For this review, take the finished solid that the model builds, in its own axes (mm). A direction names the side the tool comes from. Give positions to 0.01 mm unless a question says otherwise; leave off trailing zeros. Loops run counter-clockwise (first coordinate to the right, second up) from the corner with the lowest first, then second, coordinate; pieces in that order, holes last. Notation, with made-up numbers: M -7,65 L 28,65 A18 ccw 28,77 Z; hole C 72,-9 d8. An arc over 180 degrees is marked long. Use CSV: the item, a comma, the result in double quotes. Start each with the question number.
1. Take a section at C-C, the plane y = 44. Write out the cut boundary in (x, z), and give its area (3 significant figures).
2. Insertion check: P1, Ø2.5, axis at x = 4.76, y = -11.56, coming from the -Z side; P2, Ø6, axis at x = 11, y = 50.86, coming from the -Z side; P3, Ø3, axis at x = 37, z = 70, coming from the -Y side; P4, Ø5, axis at y = 14, z = 74.5, coming from the +X side. Each pin has a flat end and moves straight along its axis. Give the tip position at first contact, or say it passes through.
3. Tool access review of faces 3 (the face through (-6, -11, 75.5)), 4 (the face through (6.146, -11.121, 72.712)), 5 (the face through (0, -5, 70)): name each direction out of +Z, -Z, +X, -X, +Y, -Y from which nothing blocks a thin tool from reaching the whole face with its end or side.
4. The part is to be moulded in two halves that separate along X. For faces 1 (the face through (28, 1, 70)), 2 (the face through (9.214, -52.229, 73.944)), say which applies: pulls with the +X half, pulls with the -X half, needs draft (parallel to the pull), parting line crosses it, or undercut.
5. Take a section at D-D, the plane x = -36.5. Write out the cut boundary in (y, z), and give its area (3 significant figures).
6. Take a section at B-B, the plane z = 72. State how many separate pieces and enclosed holes the cut face has, and give its area (3 significant figures).
7. To check wall thickness, follow line 1 (Y direction, x = -11, z = 76.25); line 2 (Y direction, x = -11.5, z = 71.75); line 3 (Z direction, x = 26, y = -57.5). State the ranges of each line that lie inside material, in increasing order. Write a range as [from, to].
8. Take a section at A-A, the plane x = 0. Write out the cut boundary in (y, z).
from build123d import *

# Parameters (mm, degrees)
DISCO_START                         = 70
SK_DISCO_R                          = 65
DISCO_DEPTH                         = 8
CENTRADOR_ARANDELA_EJE_51110_START  = 67
SK_CENTRADOR_ARANDELA_EJE_51110_R   = 24.9
SK_CENTRADOR_ARANDELA_EJE_51110_R_2 = 23
CENTRADOR_ARANDELA_EJE_51110_DEPTH  = 3
PASANTES_M2_5_ROTOR_J1_START        = 70
SK_PASANTES_M2_5_ROTOR_J1_R         = 1.45
PASANTES_M2_5_ROTOR_J1_DEPTH        = 8
CAJAS_M2_5_START                    = 75.5
SK_CAJAS_M2_5_R                     = 2.75
CAJAS_M2_5_DEPTH                    = 2.5
PASO_CABLE_START                    = 70
SK_PASO_CABLE_R                     = 3
PASO_CABLE_DEPTH                    = 8
PASANTES_M4_ANGULOS_START           = 70
SK_PASANTES_M4_ANGULOS_R            = 2.25
PASANTES_M4_ANGULOS_DEPTH           = 8


with BuildPart() as part:
    # Sk_Disco → Disco (new body)
    with BuildSketch(Plane.XY.offset(DISCO_START)):
        Circle(SK_DISCO_R)
    extrude(amount=DISCO_DEPTH)

    # Sk_Centrador_arandela_eje_51110 → Centrador_arandela_eje_51110 (add)
    with BuildSketch(Plane.XY.offset(CENTRADOR_ARANDELA_EJE_51110_START)):
        Circle(SK_CENTRADOR_ARANDELA_EJE_51110_R)
        Circle(SK_CENTRADOR_ARANDELA_EJE_51110_R_2, mode=Mode.SUBTRACT)
    extrude(amount=CENTRADOR_ARANDELA_EJE_51110_DEPTH)

    # Sk_Pasantes_M2-5_rotor_J1 → Pasantes_M2-5_rotor_J1 (cut)
    with BuildSketch(Plane.XY.offset(PASANTES_M2_5_ROTOR_J1_START)):
        with Locations((12.390194253, -1.653204878)):
            Circle(SK_PASANTES_M2_5_ROTOR_J1_R)
        with Locations((7.626814549, 9.903620542)):
            Circle(SK_PASANTES_M2_5_ROTOR_J1_R)
        with Locations((-4.763379704, 11.55682542)):
            Circle(SK_PASANTES_M2_5_ROTOR_J1_R)
        with Locations((-12.390194253, 1.653204878)):
            Circle(SK_PASANTES_M2_5_ROTOR_J1_R)
        with Locations((-7.626814549, -9.903620542)):
            Circle(SK_PASANTES_M2_5_ROTOR_J1_R)
        with Locations((4.763379704, -11.55682542)):
            Circle(SK_PASANTES_M2_5_ROTOR_J1_R)
    extrude(amount=PASANTES_M2_5_ROTOR_J1_DEPTH, mode=Mode.SUBTRACT)

    # Sk_Cajas_M2-5 → Cajas_M2-5 (cut)
    with BuildSketch(Plane.XY.offset(CAJAS_M2_5_START)):
        with Locations((12.390194253, -1.653204878)):
            Circle(SK_CAJAS_M2_5_R)
        with Locations((7.626814549, 9.903620542)):
            Circle(SK_CAJAS_M2_5_R)
        with Locations((-4.763379704, 11.55682542)):
            Circle(SK_CAJAS_M2_5_R)
        with Locations((-12.390194253, 1.653204878)):
            Circle(SK_CAJAS_M2_5_R)
        with Locations((-7.626814549, -9.903620542)):
            Circle(SK_CAJAS_M2_5_R)
        with Locations((4.763379704, -11.55682542)):
            Circle(SK_CAJAS_M2_5_R)
    extrude(amount=CAJAS_M2_5_DEPTH, mode=Mode.SUBTRACT)

    # Sk_Paso_cable → Paso_cable (cut)
    with BuildSketch(Plane.XY.offset(PASO_CABLE_START)):
        Circle(SK_PASO_CABLE_R)
    extrude(amount=PASO_CABLE_DEPTH, mode=Mode.SUBTRACT)

    # Sk_Pasantes_M4_angulos → Pasantes_M4_angulos (cut)
    with BuildSketch(Plane.XY.offset(PASANTES_M4_ANGULOS_START)):
        with Locations((-11, -50.86)):
            Circle(SK_PASANTES_M4_ANGULOS_R)
        with Locations((-11, 50.86)):
            Circle(SK_PASANTES_M4_ANGULOS_R)
        with Locations((11, -50.86)):
            Circle(SK_PASANTES_M4_ANGULOS_R)
        with Locations((11, 50.86)):
            Circle(SK_PASANTES_M4_ANGULOS_R)
    extrude(amount=PASANTES_M4_ANGULOS_DEPTH, mode=Mode.SUBTRACT)


solid = part.part
Result set:
1,outline,"M -47.84,70 L 47.84,70 L 47.84,78 L -47.84,78 Z"
1,area,"765 mm2"
2,P1,"through"
2,P2,"z = 70"
2,P3,"y = -54.45"
2,P4,"x = 63.97"
3,face 3,"+Z"
3,face 4,"+Z, -Z"
3,face 5,"-Z"
4,face 1,"needs draft"
4,face 2,"undercut"
5,outline,"M -53.78,70 L 53.78,70 L 53.78,78 L -53.78,78 Z"
5,area,"861 mm2"
6,separate pieces,"1"
6,enclosed holes,"11"
6,area,"13,100 mm2"
7,line 1,"[-64.06, -53.11], [-48.61, -0.72], [4.03, 48.61], [53.11, 64.06]"
7,line 2,"[-63.97, -53.05], [-48.67, 0.51], [2.8, 48.67], [53.05, 63.97]"
7,line 3,"[70, 78]"
8,outline,"M -65,70 L -24.9,70 L -24.9,67 L -23,67 L -23,70 L -3,70 L -3,78 L -65,78 Z; M 3,70 L 23,70 L 23,67 L 24.9,67 L 24.9,70 L 65,70 L 65,78 L 3,78 Z"
